from build123d import *

# Parameters (mm, degrees)
SKETCH_1_W          = 17.8
SKETCH_1_H          = 8.8
SKETCH_1_W_2        = 15.8
SKETCH_1_H_2        = 6.8
EXTRUDE_1_DEPTH     = 2.5
EXTRUDE_2_DEPTH     = 1
EXTRUDE_2_TAPER     = 25
CUT_EXTRUDE_1_REACH = 5.5
SKETCH_3_R          = 1.25


with BuildPart() as part:
    # 草图1 → 凸台-拉伸1 (new body)
    with BuildSketch(Plane.XY):
        with Locations((0.435, 25.5)):
            Rectangle(SKETCH_1_W, SKETCH_1_H)
        with Locations((0.435, 25.5)):
            Rectangle(SKETCH_1_W_2, SKETCH_1_H_2, mode=Mode.SUBTRACT)
    extrude(amount=-EXTRUDE_1_DEPTH)

    # 草图2 → 凸台-拉伸2 (add)
    with BuildSketch(Plane.XY):
        with BuildLine():
            Line((10.835, 21.6), (10.835, 29.4))
            ThreePointArc((10.835, 29.4), (10.249213562, 30.814213562), (8.835, 31.4))
            Line((8.835, 31.4), (-7.965, 31.4))
            ThreePointArc((-7.965, 31.4), (-9.379213562, 30.814213562), (-9.965, 29.4))
            Line((-9.965, 29.4), (-9.965, 21.6))
            ThreePointArc((-9.965, 21.6), (-9.379213562, 20.185786438), (-7.965, 19.6))
            Line((-7.965, 19.6), (8.835, 19.6))
            ThreePointArc((8.835, 19.6), (10.249213562, 20.185786438), (10.835, 21.6))
        make_face()
    extrude(amount=EXTRUDE_2_DEPTH, taper=EXTRUDE_2_TAPER)

    # 草图3 → 切除-拉伸1 (cut, up to next)
    with BuildSketch(Plane.XY.offset(1), mode=Mode.PRIVATE) as cut_extrude_1_sk1:
        with Locations((0.435, 25.5)):
            Circle(SKETCH_3_R)
    cut_extrude_1_tool1 = extrude(cut_extrude_1_sk1.sketch, amount=-CUT_EXTRUDE_1_REACH, mode=Mode.PRIVATE) & part.part
    add(cut_extrude_1_tool1.solids().sort_by_distance((0.435, 25.5, 1))[0], mode=Mode.SUBTRACT)
    # 草图3 → 切除-拉伸1 (cut, up to next)
    with BuildSketch(Plane.XY.offset(1), mode=Mode.PRIVATE) as cut_extrude_1_sk2:
        with Locations((-3.565, 25.5)):
            Circle(SKETCH_3_R)
    cut_extrude_1_tool2 = extrude(cut_extrude_1_sk2.sketch, amount=-CUT_EXTRUDE_1_REACH, mode=Mode.PRIVATE) & part.part
    add(cut_extrude_1_tool2.solids().sort_by_distance((-3.565, 25.5, 1))[0], mode=Mode.SUBTRACT)
    # 草图3 → 切除-拉伸1 (cut, up to next)
    with BuildSketch(Plane.XY.offset(1), mode=Mode.PRIVATE) as cut_extrude_1_sk3:
        with Locations((4.435, 25.5)):
            Circle(SKETCH_3_R)
    cut_extrude_1_tool3 = extrude(cut_extrude_1_sk3.sketch, amount=-CUT_EXTRUDE_1_REACH, mode=Mode.PRIVATE) & part.part
    add(cut_extrude_1_tool3.solids().sort_by_distance((4.435, 25.5, 1))[0], mode=Mode.SUBTRACT)


solid = part.part
For this review, take the finished solid that the model builds, in its own axes (mm). A direction names the side the tool comes from. Round coordinates to 2 decimals unless told otherwise and drop trailing zeros. Loops run counter-clockwise (first coordinate to the right, second up) from the corner with the lowest first, then second, coordinate; pieces in that order, holes last. Notation, with made-up numbers: (87, 39) - (109, 39) arc R33 cw to (109, 69) - close; hole circle Ø4 at (48, -22). An arc over 180 degrees is marked (long way). One line per item, written item: value. Start each with the question number.
Item 1: For L1, parallel to Y at x = -0.75, z = -1.45; L2, parallel to X at y = 24.5, z = -2.1 (3 decimals); L3, parallel to Z at x = 1.75, y = 26.5, list the stretches that pass through material, from the lowest coordinate up.
Item 2: Take a section at B-B (y = 25.5). Give the boundary of the cut face in (x, z) (3 decimals), plus the area to 3 significant figures.
Item 3: Clearance check with flat-ended pins moving along their axes: pin 1 Ø0.8 at (y, z) = (25.5, -2) entering from +X (3 decimals); pin 2 Ø0.8 at (x, z) = (3.5, -0.5) entering from +Y; pin 3 Ø3 at (x, y) = (0.435, 25.5) entering from -Z. State where each tip first meets the part, or that it passes through.
Item 4: For faces 1 (the flat face through (-7.465, 25, -1)), 2 (the flat face through (0, 21.1, -1)), 3 (the flat face through (0, 29.9, -1)), 4 (the flat face through (9.335, 25, -1)), 5 (the flat face through (-8.465, 25, -1)), list the 3-axis set-ups (+Z, -Z, +X, -X, +Y, -Y) from which the entire face can be reached by the end or side of a thin tool; tool diameter is ignored.
Item 5: Take a section at C-C (z = -2.3). Give the boundary of the cut face in (x, y) (3 decimals).
Item 6: Take a section at D-D (x = -7.25). Give the boundary of the cut face in (y, z), plus the area to 3 significant figures.
Item 7: Take a section at A-A (x = 5.25). Give the boundary of the cut face in (y, z).
Answer below:
1. L1: y = 21.1 to 22.1, 28.9 to 29.9
1. L2: x = -8.465 to -7.465, 8.335 to 9.335
1. L3: z = 0 to 1
2. outline: (-9.965, 0) - (-8.465, 0) - (-8.465, -2.5) - (-7.465, -2.5) - (-7.465, 0) - (-4.815, 0) - (-4.815, 1) - (-9.499, 1) - close; (-2.315, 0) - (-0.815, 0) - (-0.815, 1) - (-2.315, 1) - close; (1.685, 0) - (3.185, 0) - (3.185, 1) - (1.685, 1) - close; (5.685, 0) - (8.335, 0) - (8.335, -2.5) - (9.335, -2.5) - (9.335, 0) - (10.835, 0) - (10.369, 1) - (5.685, 1) - close
2. area: 17.8 mm2
3. pin 1: stops at x = 9.335
3. pin 2: stops at y = 29.9
3. pin 3: stops at z = 0
4. face 1: -Z
4. face 2: -Z, +X, -X, -Y
4. face 3: -Z, +X, -X, +Y
4. face 4: -Z, +X, +Y, -Y
4. face 5: -Z, -X, +Y, -Y
5. outline: (-8.465, 21.1) - (9.335, 21.1) - (9.335, 29.9) - (-8.465, 29.9) - close; hole (-7.465, 22.1) - (8.335, 22.1) - (8.335, 28.9) - (-7.465, 28.9) - close
6. outline: (19.6, 0) - (21.1, 0) - (21.1, -2.5) - (22.1, -2.5) - (22.1, 0) - (28.9, 0) - (28.9, -2.5) - (29.9, -2.5) - (29.9, 0) - (31.4, 0) - (30.93, 1) - (20.07, 1) - close
6. area: 16.3 mm2
7. outline: (19.6, 0) - (21.1, 0) - (21.1, -2.5) - (22.1, -2.5) - (22.1, 0) - (24.55, 0) - (24.55, 1) - (20.07, 1) - close; (26.45, 0) - (28.9, 0) - (28.9, -2.5) - (29.9, -2.5) - (29.9, 0) - (31.4, 0) - (30.93, 1) - (26.45, 1) - close
